The model under review builds one solid part; all positions refer to its coordinate system, in mm. A direction names the side the tool comes from. Round coordinates to 2 decimals unless told otherwise and drop trailing zeros. Loops run counter-clockwise (first coordinate to the right, second up) from the corner with the lowest first, then second, coordinate; pieces in that order, holes last. Notation, with made-up numbers: (82, 64.5) -> (99, 64.5) arc R28 ccw to (99, 85.5) -> close; hole circle Ø10 at (41, 75.25). An arc over 180 degrees is marked (long way). Use a Markdown table: item, result. Add a question column.
1) Consider section D-D on x = -3.25. Give the boundary of the cut face in (y, z).
2) Insertion check: pin 1 (1 mm diameter, centred on y = 0.5, z = 1.5, fed in from +X); pin 2 (1.5 mm diameter, centred on y = 2.5, z = -2.5, fed in from -X); pin 3 (1.5 mm diameter, centred on x = 6, z = -2.5, fed in from -Y); pin 4 (1.5 mm diameter, centred on y = 1, z = 2, fed in from -X). Each pin has a flat end and moves straight along its axis. Give the tip position at first contact, or say it passes through.
3) Consider section C-C on y = 5.2. Give the boundary of the cut face in (x, z).
4) For faces 1 (the flat face through (7, 4.5, -2)), 2 (the cylindrical face through (7.154, 0.74, -2.253)), list the 3-axis set-ups (+Z, -Z, +X, -X, +Y, -Y) from which the entire face can be reached by the end or side of a thin tool; tool diameter is ignored.
5) Consider section B-B on x = 0. Give the boundary of the cut face in (y, z), plus the area to 3 significant figures.
6) Wall thickness on probe 1 along Z at (x, y) = (0, 1.3); probe 2 along Z at (x, y) = (0, 2.2); probe 3 along Y at (x, z) = (2, -7): over which ranges is each line inside the solid? List them lowest first.
7) Consider section A-A on z = 0. Give the boundary of the cut face in (x, y).
8) Mouldability with a two-part tool opening along X and no side actions: class faces 3 (the flat face through (3.2, 6, -0.1)), 4 (the cylindrical face through (2.681, 3.021, -6.466)), 5 (the cylindrical face through (-3, 3, 0)) as released by +X, released by -X, zero draft, split by the parting line, or undercut.
from build123d import *

# Parameters (mm, degrees)
SKETCH1_R           = 7.5
SKETCH1_R_2         = 3
BOSS_EXTRUDE1_DEPTH = 6
SKETCH2_W           = 0.5
SKETCH2_H           = 3


with BuildPart() as part:
    # Sketch1 → Boss-Extrude1 (new body)
    with BuildSketch(Plane(origin=(0, 0, 0), x_dir=(1, 0, 0), z_dir=(0, 1, 0))):
        Circle(SKETCH1_R)
        Circle(SKETCH1_R_2, mode=Mode.SUBTRACT)
    extrude(amount=BOSS_EXTRUDE1_DEPTH)

    # Sketch2 → Cut-Revolve1 (revolve, cut)
    with BuildSketch(Plane(origin=(0, 0, 0), x_dir=(0, 0, -1), z_dir=(1, 0, 0))):
        with Locations((7.25, 3)):
            Rectangle(SKETCH2_W, SKETCH2_H)
    revolve(axis=Axis((0, 0, 0), (0, 1, 0)), mode=Mode.SUBTRACT)


solid = part.part
Result set:
| question | item | result |
|---|---|---|
| 1 | outline | (0, -6.76) -> (1.5, -6.76) -> (1.5, -6.2) -> (4.5, -6.2) -> (4.5, -6.76) -> (6, -6.76) -> (6, 6.76) -> (4.5, 6.76) -> (4.5, 6.2) -> (1.5, 6.2) -> (1.5, 6.76) -> (0, 6.76) -> close |
| 2 | pin 1 | x = 7.43 |
| 2 | pin 2 | x = -6.78 |
| 2 | pin 3 | y = 0 |
| 2 | pin 4 | x = -7.4 |
| 3 | outline | circle Ø15 at (0, 0); hole circle Ø6 at (0, 0) |
| 4 | face 1 | none |
| 4 | face 2 | +Y, -Y |
| 5 | outline | (0, -7.5) -> (1.5, -7.5) -> (1.5, -7) -> (4.5, -7) -> (4.5, -7.5) -> (6, -7.5) -> (6, -3) -> (0, -3) -> close; (0, 3) -> (6, 3) -> (6, 7.5) -> (4.5, 7.5) -> (4.5, 7) -> (1.5, 7) -> (1.5, 7.5) -> (0, 7.5) -> close |
| 5 | area | 51.0 mm2 |
| 6 | probe 1 | -7.5 to -3, 3 to 7.5 |
| 6 | probe 2 | -7 to -3, 3 to 7 |
| 6 | probe 3 | 0 to 1.5, 4.5 to 6 |
| 7 | outline | (-7.5, 0) -> (-3, 0) -> (-3, 6) -> (-7.5, 6) -> (-7.5, 4.5) -> (-7, 4.5) -> (-7, 1.5) -> (-7.5, 1.5) -> close; (3, 0) -> (7.5, 0) -> (7.5, 1.5) -> (7, 1.5) -> (7, 4.5) -> (7.5, 4.5) -> (7.5, 6) -> (3, 6) -> close |
| 8 | face 3 | zero draft |
| 8 | face 4 | split by the parting line |
| 8 | face 5 | undercut |
